Autodesk Inventor part; units mm, degrees
ref_plane "YZ Plane" through (0, 0, 0) normal (1, 0, 0) x (0, 1, 0)
ref_plane "XZ Plane" through (0, 0, 0) normal (0, 1, 0) x (-1, 0, 0)
ref_plane "XY Plane" through (0, 0, 0) normal (0, 0, 1) x (1, 0, 0)
sketch "Sketch1" plane through (0, 0, 0) normal (0, 0, 1) x (1, 0, 0)
  line L0 (0, 0) -> (203.2, 0)
  line L1 (101.6, 152.4) -> (101.6, 0) construction
  circle A0 centre (57.8358, 12.7) radius 3.3528
  circle A1 centre (69.088, 12.7) radius 3.3528
  circle A2 centre (57.023, 45.1866) radius 2.032
  circle A3 centre (62.865, 45.1866) radius 2.54
  circle A4 centre (62.865, 63.5) radius 5.5626
  line L2 (62.865, 0) -> (62.865, 138.1252) construction
  circle A5 centre (62.865, 91.6686) radius 5.5626
  circle A6 centre (62.865, 117.0686) radius 5.5626
  circle A7 centre (69.85, 134.0866) radius 2.54
  circle A8 centre (64.008, 134.0866) radius 2.032
  circle A9 centre (101.6, 63.5) radius 14.2875
  circle A10 centre (101.6, 104.2162) radius 11.1125
  line L3 (0, 0) -> (0, 254) construction
  line L4 (203.2, 0) -> (203.2, 254) construction
  line L5 (0, 254) -> (203.2, 254) construction
  line L6 (120.9294, 254) -> (124.1044, 254) construction
  circle A11 centre (145.3642, 12.7) radius 3.3528
  circle A12 centre (134.112, 12.7) radius 3.3528
  circle A13 centre (146.177, 45.1866) radius 2.032
  circle A14 centre (140.335, 45.1866) radius 2.54
  circle A15 centre (140.335, 63.5) radius 5.5626
  line L7 (140.335, 0) -> (140.335, 138.1252) construction
  circle A16 centre (140.335, 91.6686) radius 5.5626
  circle A17 centre (140.335, 117.0686) radius 5.5626
  circle A18 centre (133.35, 134.0866) radius 2.54
  circle A19 centre (139.192, 134.0866) radius 2.032
  line L8 (0, 254) -> (0, 0)
  line L9 (0, 254) -> (203.2, 254)
  line L10 (203.2, 254) -> (203.2, 0)
  line L11 (57.8358, 12.7) -> (145.3642, 12.7) construction
  line L12 (57.023, 45.1866) -> (146.177, 45.1866) construction
  line L13 (38.1, 241.3) -> (165.1, 241.3) construction
  line L14 (165.1, 241.3) -> (165.1, 12.7) construction
  line L15 (165.1, 12.7) -> (38.1, 12.7) construction
  line L16 (38.1, 12.7) -> (38.1, 241.3) construction
  line L17 (12.7, 215.9) -> (190.5, 215.9) construction
  line L18 (190.5, 215.9) -> (190.5, 38.1) construction
  line L19 (190.5, 38.1) -> (12.7, 38.1) construction
  line L20 (12.7, 38.1) -> (12.7, 215.9) construction
  circle A20 centre (38.1, 241.3) radius 3.175
  circle A21 centre (165.1, 241.3) radius 3.175
  circle A22 centre (190.5, 215.9) radius 3.175
  circle A23 centre (12.7, 215.9) radius 3.175
  circle A24 centre (12.7, 38.1) radius 3.175
  circle A25 centre (38.1, 12.7) radius 3.175
  circle A26 centre (165.1, 12.7) radius 3.175
  circle A27 centre (190.5, 38.1) radius 3.175
  line L21 (0, 127) -> (203.2, 127) construction
  circle A28 centre (12.7, 127) radius 3.175
  circle A29 centre (190.5, 127) radius 3.175
  circle A30 centre (101.6, 241.3) radius 3.175
  circle A31 centre (12.7, 171.45) radius 3.175
  circle A32 centre (12.7, 82.55) radius 3.175
  circle A33 centre (190.5, 82.55) radius 3.175
  circle A34 centre (190.5, 171.45) radius 3.175
  circle A35 centre (88.9637, 217.6157) radius 2.1789
  circle A36 centre (150.6857, 168.5937) radius 2.1789
  point P0 (140.335, 69.0626)
  dimension "d115" = 254
  dimension "d116" = 203.2
  dimension "d130" = 77.47
  dimension "d131" = 38.735
  dimension "d133" = 31.75
  dimension "d134" = 37.592
  dimension "d135" = 38.735
  dimension "d138" = 38.735
  dimension "d149" = 12.7
  dimension "d150" = 5.08
  dimension "d151" = 4.064
  dimension "d152" = 11.1252
  dimension "d153" = 22.225
  dimension "d155" = 6.7056
  dimension "d183" = 79.0956
  dimension "d184" = 82.2706
  dimension "d185" = 101.6
  dimension "d189" = 12.7
  dimension "d190" = 38.1
  dimension "d191" = 38.1
  dimension "d192" = 12.7
  dimension "d193" = 38.1
  dimension "d194" = 12.7
  dimension "d195" = 12.7
  dimension "d196" = 38.1
  dimension "d197" = 6.35
  dimension "d198" = 6.35
  dimension "d199" = 6.35
  dimension "d200" = 6.35
  dimension "d201" = 6.35
  dimension "d202" = 6.35
  dimension "d203" = 6.35
  dimension "d204" = 6.35
  dimension "d205" = 6.35
  dimension "d206" = 6.35
  dimension "d207" = 6.35
  dimension "d213" = 6.35
  dimension "d216" = 6.35
  dimension "d218" = 6.35
  dimension "d220" = 6.35
  dimension "d225" = 177.8
  dimension "d226" = 44.45
  dimension "d227" = 44.45
  dimension "d228" = 44.45
  dimension "d229" = 44.45
  dimension "d230" = 44.45
  dimension "d231" = 44.45
  dimension "d241" = 63.5
  dimension "d242" = 40.7162
  dimension "d250" = 18.3134
  dimension "d251" = 25.4
  dimension "d252" = 17.018
  dimension "d256" = 63.5
extrude "Extrusion2" add sketch "Sketch1" along normal blind 3 contours L8 L9 L10 L0 | A35 | A36
hole "Hole4" at (132.461, 167.009, 0) at (70.739, 216.031, 0) at (153.0223, 207.5093, 0) at (153.0223, 197.3493, 0) at (50.0253, 207.5093, 0) at (50.0253, 197.3493, 0) direction (0, 0, 1) diameter 4.3688 depth 3 tip angle 118
equation "\"d191\" = d190"
equation "\"d192\" = d189"
equation "\"d193\" = d190"
equation "\"d194\" = d189"
equation "\"d195\" = d189"
equation "\"d196\" = d190"
equation "\"d226\" = 0.25 * d225"
equation "\"d228\" = 0.25 * d225"
equation "\"d229\" = d226"
equation "\"d230\" = d226"
properties part number "CustomAM-2230"
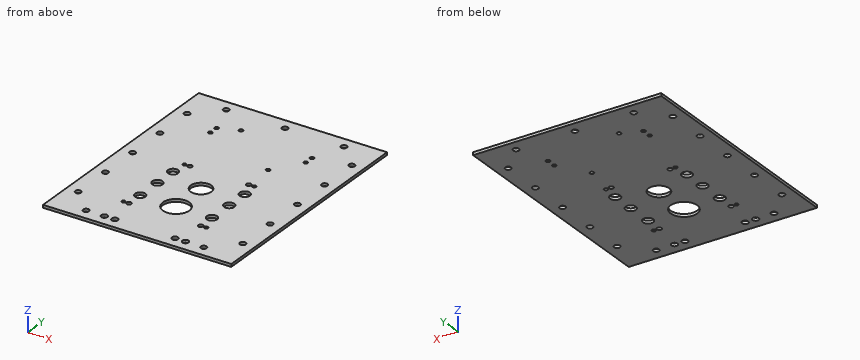
Model file for the job. Use its own axes, mm. Coordinates: 2 decimals unless noted, no trailing zeros. Write each loop counter-clockwise with the first axis right and the second up, starting at its lowest first coordinate (ties: lowest second). Pieces come first, ordered by that corner, then holes. Notation, with made-up numbers: (-25.75, 23.5) -> (-15.75, 23.5) arc R29 ccw to (-15.75, 61.5) -> close; hole circle Ø11 at (56, 25). An arc over 180 degrees is marked (long way). One line per item, written item: value. Start each with the question number.
1) Flat gauge pin, fed straight in: pin 1 Ø4.5 at (x, y) = (139.19, 134.09) entering from -Z. Where does the tip first touch, or does it go through?
2) Slice it at A-A on y = 127. Write the cut outline in (x, z) (3 decimals).
3) Slice it at D-D on y = 100.5. Write the cut outline in (x, z), then the cut area to 3 significant figures.
4) Slice it at B-B on x = 101.6. Write the cut outline in (y, z) (1 decimal).
5) Slice it at C-C on y = 12.7. Write the cut outline in (x, z) (3 decimals), then the cut area to 3 significant figures.
6) Probe probe 1 along X at (y, z) = (207, 1.05); probe 2 along Y at (x, z) = (101.6, 2.2) (1 decimal); probe 3 along X at (y, z) = (89, 2.6). List the from-to ranges inside material, lowest first.
Answers follow:
1. pin 1: z = 0
2. outline: (0, 0) -> (9.525, 0) -> (9.525, 3) -> (0, 3) -> close; (15.875, 0) -> (187.325, 0) -> (187.325, 3) -> (15.875, 3) -> close; (193.675, 0) -> (203.2, 0) -> (203.2, 3) -> (193.675, 3) -> close
3. outline: (0, 0) -> (91.13, 0) -> (91.13, 3) -> (0, 3) -> close; (112.07, 0) -> (203.2, 0) -> (203.2, 3) -> (112.07, 3) -> close
3. area: 547 mm2
4. outline: (0, 0) -> (49.2, 0) -> (49.2, 3) -> (0, 3) -> close; (77.8, 0) -> (93.1, 0) -> (93.1, 3) -> (77.8, 3) -> close; (115.3, 0) -> (238.1, 0) -> (238.1, 3) -> (115.3, 3) -> close; (244.5, 0) -> (254, 0) -> (254, 3) -> (244.5, 3) -> close
5. outline: (0, 0) -> (34.925, 0) -> (34.925, 3) -> (0, 3) -> close; (41.275, 0) -> (54.483, 0) -> (54.483, 3) -> (41.275, 3) -> close; (61.189, 0) -> (65.735, 0) -> (65.735, 3) -> (61.189, 3) -> close; (72.441, 0) -> (130.759, 0) -> (130.759, 3) -> (72.441, 3) -> close; (137.465, 0) -> (142.011, 0) -> (142.011, 3) -> (137.465, 3) -> close; (148.717, 0) -> (161.925, 0) -> (161.925, 3) -> (148.717, 3) -> close; (168.275, 0) -> (203.2, 0) -> (203.2, 3) -> (168.275, 3) -> close
5. area: 491 mm2
6. probe 1: 0 to 47.9, 52.15 to 150.9, 155.15 to 203.2
6. probe 2: 0 to 49.2, 77.8 to 93.1, 115.3 to 238.1, 244.5 to 254
6. probe 3: 0 to 57.98, 67.75 to 135.45, 145.22 to 203.2
